```python
from build123d import *

# Parameters (mm, degrees)
PAD_DEPTH = 4
FILLET_R  = 1


with BuildPart() as part:
    # Sketch → Pad (new body)
    with BuildSketch(Plane.XY):
        Polygon((0, 0), (150, 0), (75, 75), align=None)
    extrude(amount=PAD_DEPTH)

    # Fillet
    fillet_edges = [part.edges().sort_by_distance(p)[0] for p in [
        (0, 0, 2),
        (150, 0, 2),
        (75, 0, 0),
        (75, 0, 4),
        (75, 75, 2),
        (112.5, 37.5, 0),
        (112.5, 37.5, 4),
        (37.5, 37.5, 0),
        (37.5, 37.5, 4),
    ]]
    fillet(fillet_edges, radius=FILLET_R)


solid = part.part
```
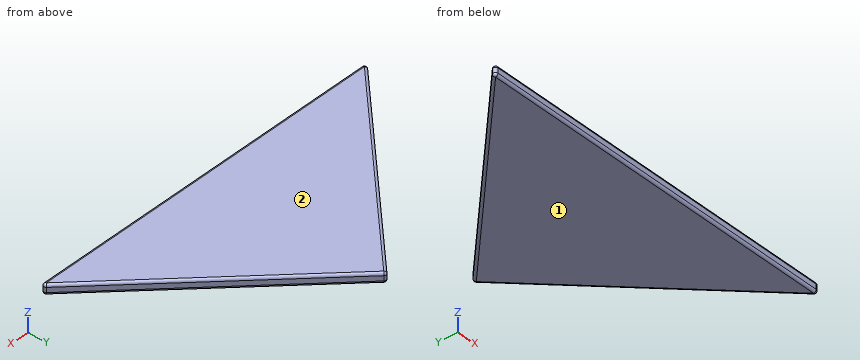
Verification items for the finished model (mm, model axes). Face numbers are marked on the shaded views. Coordinates: 2 decimals unless noted, no trailing zeros. Put each result on its own line as item: value. Start each with the question number.
1) Release check for a two-part mould opening along Z. For the marked faces 1 and 2 record: pulls with the +Z half, pulls with the -Z half, needs draft (parallel to the pull), parting line crosses it, or undercut.
2) Material ranges on L1, parallel to X at y = 67, z = 2; L2, parallel to Y at x = 40, z = 0.6; L3, parallel to X at y = 25.5, z = 1.3, recorded low to high.
3) Go/stop test with flat-tipped pins: pin 1 (12 mm diameter, centred on x = 99.5, y = 22.5, fed in from -Z); pin 2 (1 mm diameter, centred on y = 33.5, z = 2, fed in from +X); pin 3 (2 mm diameter, centred on y = 60.5, z = 0.5, fed in from +X); pin 4 (1.5 mm diameter, centred on x = 40, z = 2.5, fed in from +Y). Record where each tip stops, or that it passes through.
Geometry check:
1. face 1: pulls with the -Z half
1. face 2: pulls with the +Z half
2. L1: x = 67 to 83
2. L2: y = 0.08 to 39.88
2. L3: x = 25.5 to 124.5
3. pin 1: stops at z = 0
3. pin 2: stops at x = 117
3. pin 3: stops at x = 90.43
3. pin 4: stops at y = 40.75
